from build123d import *

# Parameters (mm, degrees)
SKETCH_1_R      = 80
SKETCH_1_R_2    = 3
SKETCH_1_R_3    = 2
SKETCH_1_R_4    = 2.5
SKETCH_1_R_5    = 2.039490197
EXTRUDE_1_DEPTH = 3


with BuildPart() as part:
    # ｽｹｯﾁ1 → ﾎﾞｽ - 押し出し1 (new body)
    with BuildSketch(Plane.XY):
        with Locations((2197.593788105, 1488.615324608)):
            Circle(SKETCH_1_R)
        with Locations((2197.593788105, 1488.615324608)):
            Circle(SKETCH_1_R_2, mode=Mode.SUBTRACT)
        with Locations((2187.593788105, 1558.615324608)):
            Circle(SKETCH_1_R_3, mode=Mode.SUBTRACT)
        with Locations((2141.97200984, 1532.275578646)):
            Circle(SKETCH_1_R_4, mode=Mode.SUBTRACT)
        with Locations((2207.593788105, 1558.615324608)):
            Circle(SKETCH_1_R_4, mode=Mode.SUBTRACT)
        with Locations((2131.97200984, 1514.95507057)):
            Circle(SKETCH_1_R_3, mode=Mode.SUBTRACT)
        with Locations((2131.97200984, 1462.275578646)):
            Circle(SKETCH_1_R_4, mode=Mode.SUBTRACT)
        with Locations((2141.97200984, 1444.95507057)):
            Circle(SKETCH_1_R_3, mode=Mode.SUBTRACT)
        with Locations((2178.093788105, 1437.836228836)):
            Circle(SKETCH_1_R_3, mode=Mode.SUBTRACT)
        with Locations((2187.593788105, 1418.615324608)):
            Circle(SKETCH_1_R_4, mode=Mode.SUBTRACT)
        with Locations((2207.593788105, 1418.615324608)):
            Circle(SKETCH_1_R_3, mode=Mode.SUBTRACT)
        with Locations((2253.21556637, 1444.95507057)):
            Circle(SKETCH_1_R_4, mode=Mode.SUBTRACT)
        with Locations((2263.21556637, 1462.275578646)):
            Circle(SKETCH_1_R_5, mode=Mode.SUBTRACT)
        with Locations((2263.21556637, 1514.95507057)):
            Circle(SKETCH_1_R_4, mode=Mode.SUBTRACT)
        with Locations((2253.21556637, 1532.275578646)):
            Circle(SKETCH_1_R_3, mode=Mode.SUBTRACT)
    extrude(amount=EXTRUDE_1_DEPTH)


solid = part.part
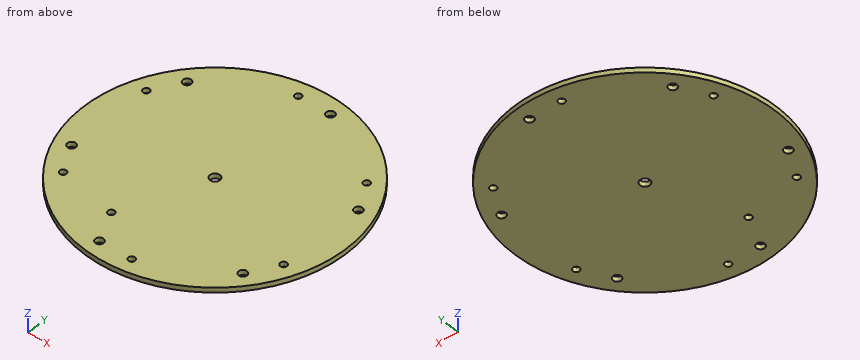
Read the model definition and answer for the solid it produces. Units are mm, in the model's axes. Coordinates: 2 decimals unless noted, no trailing zeros. Write each loop counter-clockwise with the first axis right and the second up, starting at its lowest first coordinate (ties: lowest second). Pieces come first, ordered by that corner, then holes. Notation, with made-up numbers: (-22, -5.75) -> (8, -5.75) arc R25 cw to (8, 10.25) -> close; hole circle Ø7 at (66, 60). An arc over 180 degrees is marked (long way). Return JSON: item names as keys, results as strings.
(1) Consider line 1 along X through (y, z) = (1446, 2.45); line 2 along X through (y, z) = (1516.5, 2); line 3 along Y through (x, z) = (2196.5, 0.9). Determine where each line is inside the solid, lowest interval first. Write a range as from..to.
Answers below:
{"line 1": "2129.89..2140.27, 2143.68..2250.94, 2255.49..2265.3", "line 2": "2122.61..2130.7, 2133.24..2261.25, 2265.18..2272.58", "line 3": "1408.62..1485.82, 1491.41..1568.61"}
(2) The part is cut by section C-C on x = 2215.5. Give the vertices of the cut face in (y, z).
Answers below:
{"outline": "(1410.65, 0) -> (1566.59, 0) -> (1566.59, 3) -> (1410.65, 3) -> close"}
(3) The part is cut by section A-A on z = 0.85. State how many separate pieces and enclosed holes the cut face has, then the cut area to 3 significant figures.
Answers below:
{"separate pieces": "1", "enclosed holes": "14", "area": "19,900 mm^2"}
(4) The part is cut by section B-B on y = 1424. Give the vertices of the cut face in (x, z), then the cut area to 3 significant figures.
Answers below:
{"outline": "(2150.43, 0) -> (2244.76, 0) -> (2244.76, 3) -> (2150.43, 3) -> close", "area": "283 mm^2"}
